Input: part model. Units: mm. Frame: model coordinates. Round coordinates to 2 decimals unless told otherwise and drop trailing zeros. Order: outer loops, then holes, each group sorted by start corner. A loop starts at its lowest first (then second) coordinate and runs counter-clockwise, first axis right, second up. Notation, with made-up numbers: (-23.5, -25.75) - (-1.5, -25.75) arc R23 ccw to (-1.5, -9.75) - close; hole circle Ø1 at (-25.5, 0). An arc over 180 degrees is marked (long way). One line per item, written item: value. Start each with the question number.
from build123d import *

# Parameters (mm, degrees)
ESQUISSE1_W             = 50.8
ESQUISSE1_H             = 304.8
BOSS_EXTRU_1_DEPTH      = 6.35
ESQUISSE2_R             = 2.75
ENL_V_MAT_EXTRU_1_DEPTH = 155.632604906


with BuildPart() as part:
    # Esquisse1 → Boss.-Extru.1 (new body)
    with BuildSketch(Plane.XY):
        Rectangle(ESQUISSE1_W, ESQUISSE1_H)
    extrude(amount=BOSS_EXTRU_1_DEPTH)

    # Esquisse2 → Enlèv. mat.-Extru.1 (cut, through all)
    with BuildSketch(Plane.XY.offset(6.35)):
        with Locations((12.7, 139.7)):
            Circle(ESQUISSE2_R)
        with Locations((-12.7, 139.7)):
            Circle(ESQUISSE2_R)
        with Locations(Location((12.7, -139.7, 0), (0, 0, 180))):
            Circle(ESQUISSE2_R)
        with Locations(Location((-12.7, -139.7, 0), (0, 0, 180))):
            Circle(ESQUISSE2_R)
    extrude(amount=-ENL_V_MAT_EXTRU_1_DEPTH, mode=Mode.SUBTRACT)


solid = part.part
Item 1: Pull-direction query (Y, two-part tool) for faces 1 (the face through (0, 2, 6.35)), 2 (the face through (0, -152.4, 3)), 3 (the face through (0, 152.4, 3)), 4 (the face through (13.296, -137.015, 3.219)); classes: released by +Y, released by -Y, zero draft, split by the parting line, or undercut.
Item 2: Line query: L1, parallel to Y at x = -12.7, z = 1.75; L2, parallel to X at y = 139.7, z = 5; L3, parallel to X at y = -137.5, z = 1.5. Output: solid intervals per line, ascending.
Item 3: Section query B-B on y = 139.7. Return loops of the section in (x, z).
Item 4: Section query A-A on x = -12.7. Return loops of the section in (y, z).
Item 5: First-contact query: pin 1 Ø8 at (x, y) = (-20, 38.5) entering from -Z; pin 2 Ø3.5 at (x, y) = (12.7, 139.7) entering from +Z. Flat tips, straight axial feed; report the tip coordinate or a pass-through.
Geometry results:
1. face 1: zero draft
1. face 2: released by -Y
1. face 3: released by +Y
1. face 4: undercut
2. L1: y = -152.4 to -142.45, -136.95 to 136.95, 142.45 to 152.4
2. L2: x = -25.4 to -15.45, -9.95 to 9.95, 15.45 to 25.4
2. L3: x = -25.4 to -14.35, -11.05 to 11.05, 14.35 to 25.4
3. outline: (-25.4, 0) - (-15.45, 0) - (-15.45, 6.35) - (-25.4, 6.35) - close; (-9.95, 0) - (9.95, 0) - (9.95, 6.35) - (-9.95, 6.35) - close; (15.45, 0) - (25.4, 0) - (25.4, 6.35) - (15.45, 6.35) - close
4. outline: (-152.4, 0) - (-142.45, 0) - (-142.45, 6.35) - (-152.4, 6.35) - close; (-136.95, 0) - (136.95, 0) - (136.95, 6.35) - (-136.95, 6.35) - close; (142.45, 0) - (152.4, 0) - (152.4, 6.35) - (142.45, 6.35) - close
5. pin 1: stops at z = 0
5. pin 2: passes through
